Input: part model. Units: mm. Frame: model coordinates. A direction names the side the tool comes from. Coordinates: 2 decimals unless noted, no trailing zeros. Order: outer loops, then holes, each group sorted by start corner. A loop starts at its lowest first (then second) coordinate and runs counter-clockwise, first axis right, second up. Notation, with made-up numbers: (1, 33) -> (41, 33) arc R23 cw to (41, 42) -> close; hole circle Ø3 at (-26.75, 53.25). An arc over 180 degrees is marked (long way). Use one line per item in the form item = value. Start each with the question number.
1) Pin query (flat end, axial travel): pin 1 (5 mm diameter, centred on x = 28.5, z = 8.5, fed in from -Y); pin 2 (8 mm diameter, centred on y = -9, z = 12.5, fed in from -X); pin 3 (15 mm diameter, centred on x = 16.5, y = -2, fed in from +Z). Return the tip coordinate at first contact, or that it passes through.
2) Section query B-B on y = 4. Output: boundary loops of the cut face in (x, z).
3) Ray query, line 1 along X through (y, z) = (10, 6); line 2 along Z through (x, y) = (6.5, 13); line 3 along X through (y, z) = (-10, 10.5). Return the intervals inside material, ascending.
4) Section query D-D on y = -13. Output: boundary loops of the cut face in (x, z).
5) Draft query along Z for faces 1 (the flat face through (24, -2, 0)), 2 (the flat face through (46.038, 6, 7)), 3 (the flat face through (23.6, 12.6, 3)). Return one class per face: pulls with the +Z half, pulls with the -Z half, needs draft (parallel to the pull), parting line crosses it, or undercut.
6) Section query C-C on x = 20.5. Output: boundary loops of the cut face in (y, z), then the cut area to 3 significant figures.
7) Section query A-A on z = 10.75. Output: boundary loops of the cut face in (x, y) (3 decimals), then the cut area to 3 significant figures.
8) Access query for faces 4 (the flat face through (9.44, -10.55, 7.92)), 5 (the flat face through (24.1, 12.6, 13)), 6 (the flat face through (24, 13, 14)). Directions: +Z, -Z, +X, -X, +Y, -Y. A direction counts if a zero-diameter tool reaches every point of the face in a straight line with its end or side. Return the directions, or none.
from build123d import *

# Parameters (mm, degrees)
EXTRUDE_1_DEPTH     = 2
EXTRUDE_5_DEPTH     = 12
SKETCH_3_R          = 2
EXTRUDE_6_DEPTH     = 12
CUT_EXTRUDE_1_DEPTH = 12
EXTRUDE_7_DEPTH     = 15
SKETCH_7_W          = 44.36597813
SKETCH_7_H          = 14
EXTRUDE_8_DEPTH     = 3
SKETCH_9_W          = 18.66
SKETCH_9_H          = 10
CUT_EXTRUDE_3_DEPTH = 1


with BuildPart() as part:
    # 스케치2 → 보스-돌출1 (new body)
    with BuildSketch(Plane.XY):
        Polygon((0, 0), (47.71, 0), (37.32, -17.996007891), (10.39, -17.996007891), align=None)
    extrude(amount=EXTRUDE_1_DEPTH)

    # 스케치4 → 보스-돌출5 (add)
    with BuildSketch(Plane.XY.offset(2)):
        Polygon((13.739529946, -17.996007891), (5.021540881, -2.896007891), (1.672010935, -2.896007891), (10.39, -17.996007891), align=None)
        Polygon((46.037989065, -2.896007891), (42.688459119, -2.896007891), (33.970470054, -17.996007891), (37.32, -17.996007891), align=None)
    extrude(amount=EXTRUDE_5_DEPTH)

    # 스케치3 → 보스-돌출6 (add)
    with BuildSketch(Plane.XY.offset(2)):
        with Locations(Location((15.355, -11.594084102, 0), (0, 0, 180))):
            Circle(SKETCH_3_R)
        with Locations((32.355, -11.594084102)):
            Circle(SKETCH_3_R)
    extrude(amount=EXTRUDE_6_DEPTH)

    # 스케치5 → 컷-돌출1 (cut)
    with BuildSketch(Plane.XY.offset(2)):
        Polygon((0, 0), (47.71, 0), (46.037989065, -2.896007891), (1.672010935, -2.896007891), align=None)
    extrude(amount=-CUT_EXTRUDE_1_DEPTH, mode=Mode.SUBTRACT)

    # 스케치6 → 보스-돌출7 (add)
    with BuildSketch(Plane(origin=(0, -2.896007891, 0), x_dir=(1, 0, 0), z_dir=(0, 1, 0))):
        Polygon((5.021540881, -14), (1.672010935, -14), (1.672010935, 0), (46.037989065, 0), (46.037989065, -14), (42.688459119, -14), (42.688459119, -2), (5.021540881, -2), align=None)
    extrude(amount=EXTRUDE_7_DEPTH)

    # 스케치7 → 보스-돌출8 (add)
    with BuildSketch(Plane(origin=(0, 12.103992109, 0), x_dir=(1, 0, 0), z_dir=(0, 1, 0))):
        with Locations((23.855, -7)):
            Rectangle(SKETCH_7_W, SKETCH_7_H)
    extrude(amount=EXTRUDE_8_DEPTH)

    # 스케치9 → 컷-돌출3 (cut)
    with BuildSketch(Plane.XZ.offset(-12.103992109)):
        with Locations((14.525, 8)):
            Rectangle(SKETCH_9_W, SKETCH_9_H)
        with Locations((33.185, 8)):
            Rectangle(SKETCH_9_W, SKETCH_9_H)
    extrude(amount=-CUT_EXTRUDE_3_DEPTH, mode=Mode.SUBTRACT)


solid = part.part
Answers below:
q1.pin_1 = -13.07
q1.pin_2 = 2.89
q1.pin_3 = 2
q2.outline = (1.67, 0) -> (46.04, 0) -> (46.04, 14) -> (42.69, 14) -> (42.69, 2) -> (5.02, 2) -> (5.02, 14) -> (1.67, 14) -> close
q3.line_1 = 1.67 to 5.02, 42.69 to 46.04
q3.line_2 = 0 to 3, 13 to 14
q3.line_3 = 5.77 to 9.12, 14.15 to 16.56, 31.15 to 33.56, 38.59 to 41.94
q4.outline = (7.51, 0) -> (40.2, 0) -> (40.2, 14) -> (36.85, 14) -> (36.85, 2) -> (33.78, 2) -> (33.78, 14) -> (30.93, 14) -> (30.93, 2) -> (16.78, 2) -> (16.78, 14) -> (13.93, 14) -> (13.93, 2) -> (10.86, 2) -> (10.86, 14) -> (7.51, 14) -> close
q5.face_1 = pulls with the -Z half
q5.face_2 = needs draft
q5.face_3 = undercut
q6.outline = (-18, 0) -> (15.1, 0) -> (15.1, 14) -> (12.1, 14) -> (12.1, 13) -> (13.1, 13) -> (13.1, 3) -> (12.1, 3) -> (12.1, 2) -> (-18, 2) -> close
q6.area = 92.2 mm^2
q7.outline = (1.672, -2.896) -> (10.39, -17.996) -> (13.74, -17.996) -> (5.022, -2.896) -> (5.022, 12.104) -> (5.195, 12.104) -> (5.195, 13.104) -> (42.515, 13.104) -> (42.515, 12.104) -> (42.688, 12.104) -> (42.688, -2.896) -> (33.97, -17.996) -> (37.32, -17.996) -> (46.038, -2.896) -> (46.038, 15.104) -> (1.672, 15.104) -> close; circle Ø4 at (15.355, -11.594); circle Ø4 at (32.355, -11.594)
q7.area = 323 mm^2
q8.face_4 = +Z
q8.face_5 = none
q8.face_6 = +Z, +X, -X, +Y, -Y
